```python
from build123d import *

# Parameters (mm, degrees)
SKETCH1_W            = 31.115
SKETCH1_H            = 17.145
MOTOR_BODY_DEPTH     = 30.0482
FASTENING_HOLE_DEPTH = 1.9812
SKETCH3_R            = 1.4605
SHAFT_HOLE_DEPTH     = 31.0482


with BuildPart() as part:
    # Sketch1 → Motor Body (new body)
    with BuildSketch(Plane.XY):
        Rectangle(SKETCH1_W, SKETCH1_H)
    extrude(amount=MOTOR_BODY_DEPTH)

    # Sketch2 → Fastening hole (add)
    with BuildSketch(Plane.XZ.offset(8.5725)):
        with BuildLine():
            Line((-0.8763, -7.4676), (5.5245, -7.4676))
            ThreePointArc((5.5245, -7.4676), (6.422525612, -7.095625612), (6.7945, -6.1976))
            Line((6.7945, -6.1976), (6.7945, 0))
            Line((6.7945, 0), (-2.1463, 0))
            Line((-2.1463, 0), (-2.1463, -6.1976))
            ThreePointArc((-2.1463, -6.1976), (-1.774325612, -7.095625612), (-0.8763, -7.4676))
        make_face()
        with BuildLine():
            Line((0.6858, -5.4356), (3.8862, -5.4356))
            ThreePointArc((3.8862, -5.4356), (4.784225612, -5.063625612), (5.1562, -4.1656))
            Line((5.1562, -4.1656), (5.1562, -3.5306))
            ThreePointArc((5.1562, -3.5306), (4.784225612, -2.632574388), (3.8862, -2.2606))
            Line((3.8862, -2.2606), (0.6858, -2.2606))
            ThreePointArc((0.6858, -2.2606), (-0.212225612, -2.632574388), (-0.5842, -3.5306))
            Line((-0.5842, -3.5306), (-0.5842, -4.1656))
            ThreePointArc((-0.5842, -4.1656), (-0.212225612, -5.063625612), (0.6858, -5.4356))
        make_face(mode=Mode.SUBTRACT)
    extrude(amount=-FASTENING_HOLE_DEPTH)

    # Sketch3 → Shaft hole (cut, through all)
    with BuildSketch(Plane(origin=(0, 0, 0), x_dir=(-1, 0, 0), z_dir=(0, 0, -1))):
        with Locations((11.0109, 3.4925)):
            Circle(SKETCH3_R)
    extrude(amount=-SHAFT_HOLE_DEPTH, mode=Mode.SUBTRACT)


solid = part.part
```
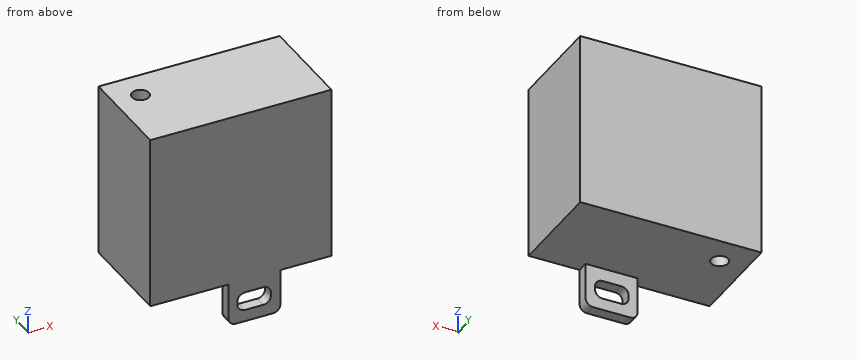
Verification items for the finished model (mm, model axes). Give positions to 0.01 mm unless a question says otherwise; leave off trailing zeros. Loops run counter-clockwise (first coordinate to the right, second up) from the corner with the lowest first, then second, coordinate; pieces in that order, holes last.
1. Section check C-C, the plane x = -9. Enter the section's corners in (y, z).
2. Thickness scan on line 1 (Z direction, x = 6.5, y = 1.25); line 2 (X direction, y = 4.5, z = 20.5); line 3 (Y direction, x = -11.5, z = 3). Record the ranges inside material, lowest first.
3. Section check D-D, the plane y = -1. Enter the section's corners in (x, z), then the cut area to 3 significant figures.
4. Section check B-B, the plane y = -7.5. Enter the section's corners in (x, z).
5. Go/stop test with flat-tipped pins: pin 1 Ø0.6 at (y, z) = (-7, -4) entering from -X; pin 2 Ø2 at (x, z) = (2.5, -5) entering from +Y; pin 3 Ø8.5 at (x, y) = (-4.5, 1.5) entering from -Z. Record where each tip stops, or that it passes through.
6. Section check A-A, the plane x = 2.5. Enter the section's corners in (y, z).
Geometry says:
1. outline: (-8.57, 0) - (8.57, 0) - (8.57, 30.05) - (-8.57, 30.05) - close
2. line 1: z = 0 to 30.05
2. line 2: x = -15.56 to -12.07, -9.95 to 15.56
2. line 3: y = -8.57 to 2.12, 4.87 to 8.57
3. outline: (-15.56, 0) - (15.56, 0) - (15.56, 30.05) - (-15.56, 30.05) - close
3. area: 935 mm2
4. outline: (-15.56, 0) - (-2.15, 0) - (-2.15, -6.2) arc R1.27 ccw to (-0.88, -7.47) - (5.52, -7.47) arc R1.27 ccw to (6.79, -6.2) - (6.79, 0) - (15.56, 0) - (15.56, 30.05) - (-15.56, 30.05) - close; hole (-0.58, -4.17) arc R1.27 ccw to (0.69, -5.44) - (3.89, -5.44) arc R1.27 ccw to (5.16, -4.17) - (5.16, -3.53) arc R1.27 ccw to (3.89, -2.26) - (0.69, -2.26) arc R1.27 ccw to (-0.58, -3.53) - close
5. pin 1: stops at x = -2.15
5. pin 2: stops at y = -6.59
5. pin 3: stops at z = 0
6. outline: (-8.57, -7.47) - (-6.59, -7.47) - (-6.59, -5.44) - (-8.57, -5.44) - close; (-8.57, -2.26) - (-6.59, -2.26) - (-6.59, 0) - (8.57, 0) - (8.57, 30.05) - (-8.57, 30.05) - close
